from build123d import *

# Parameters (mm, degrees)
BOSS_EXTRU_1_DEPTH      = 60
ESQUISSE2_W             = 41
ESQUISSE2_H             = 41
ENL_V_MAT_EXTRU_1_DEPTH = 50
CONG_1_R                = 4
ESQUISSE4_R             = 3.5
ENL_V_MAT_EXTRU_2_DEPTH = 61
ESQUISSE6_R             = 2
ENL_V_MAT_EXTRU_4_DEPTH = 81
ESQUISSE7_R             = 1.35
ENL_V_MAT_EXTRU_5_DEPTH = 11


with BuildPart() as part:
    # Esquisse1 → Boss.-Extru.1 (new body)
    with BuildSketch(Plane.XY):
        Polygon((0, 0), (-60, 0), (-60, -54), (-80, -54), (-80, -60), (20, -60), (20, -54), (0, -54), align=None)
    extrude(amount=-BOSS_EXTRU_1_DEPTH)

    # Esquisse2 → Enlèv. mat.-Extru.1 (cut)
    with BuildSketch(Plane.XY):
        with Locations((-30, -30)):
            Rectangle(ESQUISSE2_W, ESQUISSE2_H)
    extrude(amount=-ENL_V_MAT_EXTRU_1_DEPTH, mode=Mode.SUBTRACT)

    # Congé1
    cong_1_edges = [part.edges().sort_by_distance(p)[0] for p in [
        (-50.5, -50.5, -25),
        (-50.5, -9.5, -25),
        (-9.5, -9.5, -25),
        (-9.5, -50.5, -25),
    ]]
    fillet(cong_1_edges, radius=CONG_1_R)

    # Esquisse4 → Enlèv. mat.-Extru.2 (cut, through all)
    with BuildSketch(Plane.XZ.offset(60)):
        with Locations((-70, -11.134276922)):
            Circle(ESQUISSE4_R)
        with Locations((-70, -30)):
            Circle(ESQUISSE4_R)
        with Locations((-70, -48.052106988)):
            Circle(ESQUISSE4_R)
        with Locations((10, -48.052106988)):
            Circle(ESQUISSE4_R)
        with Locations((10, -30)):
            Circle(ESQUISSE4_R)
        with Locations((10, -11.134276922)):
            Circle(ESQUISSE4_R)
    extrude(amount=-ENL_V_MAT_EXTRU_2_DEPTH, mode=Mode.SUBTRACT)

    # Esquisse6 → Enlèv. mat.-Extru.4 (cut, through all)
    with BuildSketch(Plane.ZY.offset(60)):
        with Locations((-31.500403789, -18)):
            Circle(ESQUISSE6_R)
        with Locations((-31.500403789, -42)):
            Circle(ESQUISSE6_R)
    extrude(amount=-ENL_V_MAT_EXTRU_4_DEPTH, mode=Mode.SUBTRACT)

    # Esquisse7 → Enlèv. mat.-Extru.5 (cut, through all)
    with BuildSketch(Plane.XY.offset(-50)):
        with Locations((-30, -17.5)):
            Circle(ESQUISSE7_R)
    extrude(amount=-ENL_V_MAT_EXTRU_5_DEPTH, mode=Mode.SUBTRACT)


solid = part.part
Verification items for the finished model (mm, model axes). A direction names the side the tool comes from. Give positions to 0.01 mm unless a question says otherwise; leave off trailing zeros. Loops run counter-clockwise (first coordinate to the right, second up) from the corner with the lowest first, then second, coordinate; pieces in that order, holes last.
1) Draft check along X on faces 4 (the flat face through (6, -54, -30)), 5 (the flat face through (20, -57, -30)), 6 (the cylindrical face through (9.54, -57.04, -26.53)). Enter one of: pulls with the +X half, pulls with the -X half, needs draft (parallel to the pull), parting line crosses it, or undercut.
2) Sectioned sample at C-C, the plane z = -56. Enter the section's corners in (x, y), then the cut area to 3 significant figures.
3) Thickness scan on line 1 along Z through (x, y) = (10, -56); line 2 along Y through (x, z) = (-15.5, -36); line 3 along Y through (x, z) = (-58.5, -32.5). Record the ranges inside material, lowest first.
4) Sectioned sample at D-D, the plane y = -42. Enter the section's corners in (x, z), then the cut area to 3 significant figures.
5) Depth check by flat-ended pin: pin 1 Ø2.5 at (y, z) = (-42, -31.5) entering from +X; pin 2 Ø3 at (y, z) = (-11, -48) entering from +X; pin 3 Ø6.5 at (y, z) = (-18, -31.5) entering from -X; pin 4 Ø6 at (x, z) = (-66, -20.5) entering from +Y. Enter the tip coordinate at first touch or a pass-through.
6) Set-up check for faces 1 (the cylindrical face through (-55.316, -16.648, -32.974)), 2 (the flat face through (-74, -54, -30)), 3 (the cylindrical face through (-10.703, -49.359, -25.35)): record each of +Z, -Z, +X, -X, +Y, -Y from which the full face is reachable in a straight line by a thin tool's end or side.
7) Sectioned sample at B-B, the plane x = 10. Enter the section's corners in (y, z), then the cut area to 3 significant figures.
8) Sectioned sample at A-A, the plane x = -30. Enter the section's corners in (y, z), then the cut area to 3 significant figures.
Answers:
1. face 4: needs draft
1. face 5: pulls with the +X half
1. face 6: undercut
2. outline: (-80, -60) - (20, -60) - (20, -54) - (0, -54) - (0, 0) - (-60, 0) - (-60, -54) - (-80, -54) - close; hole circle Ø2.7 at (-30, -17.5)
2. area: 3,830 mm2
3. line 1: z = -60 to -51.55, -44.55 to -33.5, -26.5 to -14.63, -7.63 to 0
3. line 2: y = -60 to -50.5, -9.5 to 0
3. line 3: y = -60 to -43.73, -40.27 to -19.73, -16.27 to 0
4. outline: (-60, -60) - (0, -60) - (0, -33.5) - (-9.5, -33.5) - (-9.5, -50) - (-50.5, -50) - (-50.5, -33.5) - (-60, -33.5) - close; (-60, -29.5) - (-50.5, -29.5) - (-50.5, 0) - (-60, 0) - close; (-9.5, -29.5) - (0, -29.5) - (0, 0) - (-9.5, 0) - close
4. area: 1,470 mm2
5. pin 1: passes through
5. pin 2: stops at x = 0
5. pin 3: stops at x = -60
5. pin 4: stops at y = -54
6. face 1: +X, -X
6. face 2: +Z, -Z, -X, +Y
6. face 3: +Z
7. outline: (-60, -60) - (-54, -60) - (-54, -51.55) - (-60, -51.55) - close; (-60, -44.55) - (-54, -44.55) - (-54, -33.5) - (-60, -33.5) - close; (-60, -26.5) - (-54, -26.5) - (-54, -14.63) - (-60, -14.63) - close; (-60, -7.63) - (-54, -7.63) - (-54, 0) - (-60, 0) - close
7. area: 234 mm2
8. outline: (-60, -60) - (-18.85, -60) - (-18.85, -50) - (-50.5, -50) - (-50.5, 0) - (-60, 0) - close; (-16.15, -60) - (0, -60) - (0, 0) - (-9.5, 0) - (-9.5, -50) - (-16.15, -50) - close
8. area: 1,520 mm2
